Geometry: see drawing. Coordinates: mm, zero at the bounding-box minimum. Coordinates: 2 decimals unless noted, no trailing zeros. Order: outer loops, then holes, each group sorted by start corner. A loop starts at its lowest first (then second) coordinate and runs counter-clockwise, first axis right, second up. Notation, with made-up numbers: (-15.75, -20) -> (39.25, -20) arc R23 ccw to (39.25, 12) -> close; hole circle Ø1 at (69.5, 5.5). An arc over 180 degrees is marked (long way). Use CSV: the item, a comma, the result in double quotes. Start each with the question number.
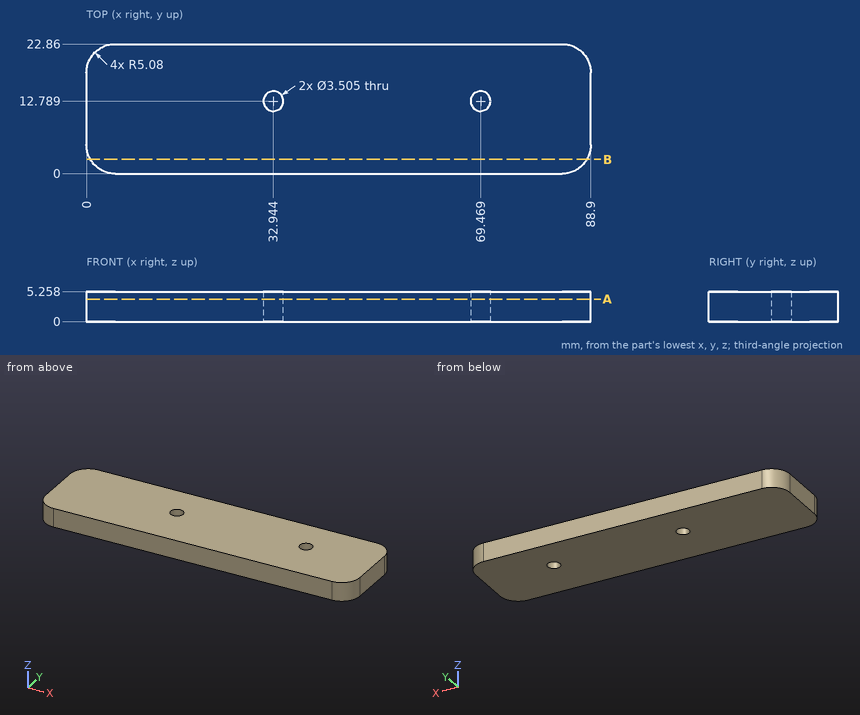
(1) First-contact query: pin 1 (4 mm diameter, centred on x = 76, y = 19.5, fed in from -Z). Flat tip, straight axial feed; report the tip coordinate or a pass-through.
(2) Section B-B (y = 2.5). Return loops of the section in (x, z).
(3) Section A-A (z = 3.95). Return loops of the section in (x, y) (1 decimal), then the cut area to 3 significant figures.
(4) Line query: line 1 (Y direction, x = 5, z = 2.65); line 2 (X direction, y = 13.75, z = 0.7) (1 decimal); line 3 (Y direction, x = 68, z = 3.5) (1 decimal). Output: solid intervals per line, ascending. Write a range as from..to.
Check sheet entries:
1,pin 1,"stops at z = 0"
2,outline,"(0.7, 0) -> (88.2, 0) -> (88.2, 5.26) -> (0.7, 5.26) -> close"
3,outline,"(0, 5.1) arc R5.1 ccw to (5.1, 0) -> (83.8, 0) arc R5.1 ccw to (88.9, 5.1) -> (88.9, 17.8) arc R5.1 ccw to (83.8, 22.9) -> (5.1, 22.9) arc R5.1 ccw to (0, 17.8) -> close; hole circle Ø3.5 at (32.9, 12.8); hole circle Ø3.5 at (69.5, 12.8)"
3,area,"1,990 mm^2"
4,line 1,"y = 0..22.86"
4,line 2,"x = 0..31.5, 34.4..68, 70.9..88.9"
4,line 3,"y = 0..11.8, 13.7..22.9"
